Build history of the part. All positions in model axes, mm. Face numbers are marked on the shaded views. A direction names the side the tool comes from. Round coordinates to 2 decimals unless told otherwise and drop trailing zeros. Write each loop counter-clockwise with the first axis right and the second up, starting at its lowest first coordinate (ties: lowest second). Pieces come first, ordered by that corner, then holes. Notation, with made-up numbers: (22, 1) - (56, 1) arc R14 ccw to (56, 13) - close; hole circle Ø3 at (59.25, 60). An arc over 180 degrees is marked (long way). Answer as a JSON object with one key per item and string values. Group by question number.
Item 1: Which spindle directions (+Z, -Z, +X, -X, +Y, -Y) get a long thin tool onto all of the face, cutting with end or side? Do the marked faces 1, 2, 3, 4 and 5. Say none if no direction does.
Item 2: Slice it at D-D, the plane z = 0. Give the number of separate pieces and of enclosed holes in the cut face, then the cut area to 3 significant figures.
Item 3: Probe line 1 (X direction, y = 0.95, z = 0); line 2 (Z direction, x = 0, y = 4.25). List the from-to ranges inside material, lowest first. Write a range as from..to.
Item 4: Slice it at A-A, the plane z = 11. List the corners of the cut face in (x, y), then the cut area to 3 significant figures.
Item 5: Slice it at B-B, the plane x = 11. List the corners of the cut face in (y, z), then the cut area to 3 significant figures.
Item 6: Flat gauge pins, fed straight in: pin 1 (6 mm diameter, centred on y = 17.5, z = 10, fed in from +X); pin 2 (5 mm diameter, centred on x = 2.5, y = 15.5, fed in from +Z); pin 3 (3 mm diameter, centred on x = -5.5, y = 4, fed in from +Z). Where does each tip first touch, or does it go through?
Item 7: Slice it at C-C, the plane y = 25. List the corners of the cut face in (x, z), then the cut area to 3 significant figures.
Item 8: Two-plate mould, pull along Y, no slides. Class the marked faces 6, 7 and 8: +Y half, -Y half, draft (parallel to the pull), parting line (faces both ways), or undercut.
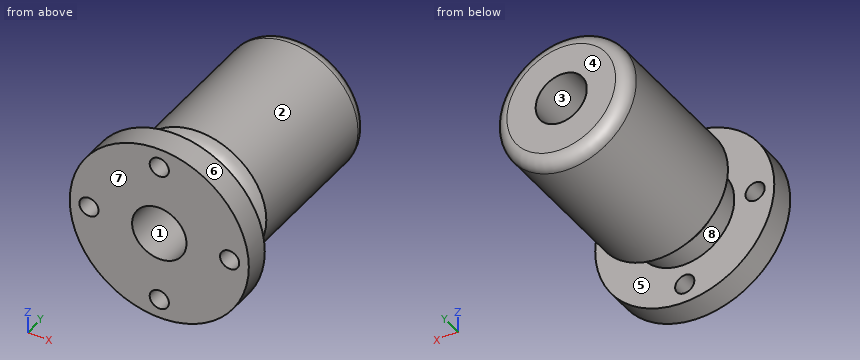
from build123d import *

# Parameters (mm, degrees)
SKETCH1_R           = 14
SKETCH1_R_2         = 1.5
SKETCH1_R_3         = 4.25
BOSS_EXTRUDE1_DEPTH = 4
SKETCH2_R           = 7.75
SKETCH2_R_2         = 4.25
BOSS_EXTRUDE2_DEPTH = 6
SKETCH3_R           = 10.5
SKETCH3_R_2         = 4
BOSS_EXTRUDE3_DEPTH = 25
FILLET1_R           = 2


with BuildPart() as part:
    # Sketch1 → Boss-Extrude1 (new body)
    with BuildSketch(Plane(origin=(0, 0, 0), x_dir=(1, 0, 0), z_dir=(0, 1, 0))):
        Circle(SKETCH1_R)
        with Locations((0, 11)):
            Circle(SKETCH1_R_2, mode=Mode.SUBTRACT)
        with Locations((0, -11)):
            Circle(SKETCH1_R_2, mode=Mode.SUBTRACT)
        with Locations((11, 0)):
            Circle(SKETCH1_R_2, mode=Mode.SUBTRACT)
        with Locations((-11, 0)):
            Circle(SKETCH1_R_2, mode=Mode.SUBTRACT)
        Circle(SKETCH1_R_3, mode=Mode.SUBTRACT)
    extrude(amount=BOSS_EXTRUDE1_DEPTH)

    # Sketch2 → Boss-Extrude2 (add)
    with BuildSketch(Plane(origin=(0, 4, 0), x_dir=(1, 0, 0), z_dir=(0, 1, 0))):
        Circle(SKETCH2_R)
        Circle(SKETCH2_R_2, mode=Mode.SUBTRACT)
    extrude(amount=BOSS_EXTRUDE2_DEPTH)



with BuildPart() as body_2:
    # Sketch3 → Boss-Extrude3 (new body)
    with BuildSketch(Plane(origin=(0, 10, 0), x_dir=(1, 0, 0), z_dir=(0, 1, 0))):
        Circle(SKETCH3_R)
        Circle(SKETCH3_R_2, mode=Mode.SUBTRACT)
    extrude(amount=BOSS_EXTRUDE3_DEPTH)


with BuildPart() as part_1:
    add(part.part)

    add(body_2.part)  # Revolve1 merges body 2
    # Sketch4 → Revolve1 (revolve)
    with BuildSketch(Plane(origin=(0, 0, 0), x_dir=(0, 0, -1), z_dir=(1, 0, 0))):
        with BuildLine():
            Line((7.75, 10), (10.5, 10))
            add(Edge.make_bspline(
                [(10.5, 10), (8.289227016, 9.506903226), (7.75, 7.304459311)],
                knots=[0, 0, 0, 1, 1, 1], degree=2))
            Line((7.75, 7.304459311), (7.75, 10))
        make_face()
    revolve(axis=Axis((0, 36.75, 0), (0, -1, 0)))

    # Fillet1
    fillet1_edges = [part_1.edges().sort_by_distance(p)[0] for p in [
        (-10.5, 35, 0),
    ]]
    fillet(fillet1_edges, radius=FILLET1_R)


solid = part_1.part
Geometry says:
{
 "1": {"face 1": "-Y", "face 2": "+Y", "face 3": "+Y, -Y", "face 4": "+Z, -Z, +X, -X, +Y", "face 5": "none"},
 "2": {"separate pieces": "4", "enclosed holes": "0", "area": "424 mm^2"},
 "3": {"line 1": "x = -14..-12.5, -9.5..-4.25, 4.25..9.5, 12.5..14", "line 2": "z = -7.75..-4.25, 4.25..7.75"},
 "4": {"outline": "(-8.66, 0) - (-1.5, 0) - (-1.5, 4) - (-8.66, 4) - close; (1.5, 0) - (8.66, 0) - (8.66, 4) - (1.5, 4) - close", "area": "57.3 mm^2"},
 "5": {"outline": "(0, -8.66) - (4, -8.66) - (4, -1.5) - (0, -1.5) - close; (0, 1.5) - (4, 1.5) - (4, 8.66) - (0, 8.66) - close", "area": "57.3 mm^2"},
 "6": {"pin 1": "stops at x = 7.83", "pin 2": "stops at z = 10.5", "pin 3": "stops at z = 13.42"},
 "7": {"outline": "circle Ø21 at (0, 0); hole circle Ø8 at (0, 0)", "area": "296 mm^2"},
 "8": {"face 6": "draft", "face 7": "-Y half", "face 8": "undercut"}
}
